```python
from build123d import *

# Parameters (mm, degrees)
SKETCH1_W                  = 101.6
SKETCH1_H                  = 177.8
BOSS_EXTRUDE1_DEPTH        = 12.7
F_10_32_TAPPED_HOLE1_D     = 4.0386
F_10_32_TAPPED_HOLE1_DEPTH = 25.4
F_10_32_TAPPED_HOLE1_TIP   = 1.213317848
SKETCH5_R                  = 12.7
SKETCH5_R_2                = 3.175
CUT_EXTRUDE1_DEPTH         = 104.175287739
SKETCH6_W                  = 61.595
SKETCH6_H                  = 61.595
CUT_EXTRUDE2_DEPTH         = 9.398
FILLET1_R                  = 3.175
SKETCH7_W                  = 67.945
SKETCH7_H                  = 67.945
CUT_EXTRUDE3_DEPTH         = 4.445
FILLET2_R                  = 3.175


with BuildPart() as part:
    # Sketch1 → Boss-Extrude1 (new body)
    with BuildSketch(Plane.XY):
        Rectangle(SKETCH1_W, SKETCH1_H)
    extrude(amount=BOSS_EXTRUDE1_DEPTH)

    # #10-32 Tapped Hole1
    with Locations(Plane(origin=(0, -88.9, 0), x_dir=(-1, 0, 0), z_dir=(0, -1, 0))):
        with Locations((31.75, -6.35), (-31.75, -6.35)):
            Hole(F_10_32_TAPPED_HOLE1_D / 2, depth=F_10_32_TAPPED_HOLE1_DEPTH)
            with Locations((0, 0, -(F_10_32_TAPPED_HOLE1_DEPTH + F_10_32_TAPPED_HOLE1_TIP / 2))):  # 118° drill point
                Cone(0, F_10_32_TAPPED_HOLE1_D / 2, F_10_32_TAPPED_HOLE1_TIP, mode=Mode.SUBTRACT)

    # Sketch5 → Cut-Extrude1 (cut, through all)
    with BuildSketch(Plane.XY.offset(12.7)):
        with Locations((0, 38.616692093)):
            Circle(SKETCH5_R)
        with Locations((-27.305, 65.921692093)):
            Circle(SKETCH5_R_2)
        with Locations((27.305, 65.921692093)):
            Circle(SKETCH5_R_2)
        with Locations((27.305, 11.311692093)):
            Circle(SKETCH5_R_2)
        with Locations((-27.305, 11.311692093)):
            Circle(SKETCH5_R_2)
    extrude(amount=-CUT_EXTRUDE1_DEPTH, mode=Mode.SUBTRACT)

    # Sketch6 → Cut-Extrude2 (cut)
    with BuildSketch(Plane(origin=(0, 0, 0), x_dir=(-1, 0, 0), z_dir=(0, 0, -1))):
        with Locations((0, 38.616692093)):
            Rectangle(SKETCH6_W, SKETCH6_H)
    extrude(amount=-CUT_EXTRUDE2_DEPTH, mode=Mode.SUBTRACT)

    # Fillet1
    fillet1_edges = [part.edges().sort_by_distance(p)[0] for p in [
        (-30.7975, 69.414192093, 4.699),
        (-30.7975, 7.819192093, 4.699),
        (30.7975, 7.819192093, 4.699),
        (30.7975, 69.414192093, 4.699),
    ]]
    fillet(fillet1_edges, radius=FILLET1_R)

    # Sketch7 → Cut-Extrude3 (cut)
    with BuildSketch(Plane(origin=(0, 0, 0), x_dir=(-1, 0, 0), z_dir=(0, 0, -1))):
        with Locations((0, 38.616692093)):
            Rectangle(SKETCH7_W, SKETCH7_H)
    extrude(amount=-CUT_EXTRUDE3_DEPTH, mode=Mode.SUBTRACT)

    # Fillet2
    fillet2_edges = [part.edges().sort_by_distance(p)[0] for p in [
        (-33.9725, 72.589192093, 2.2225),
        (-33.9725, 4.644192093, 2.2225),
        (33.9725, 4.644192093, 2.2225),
        (33.9725, 72.589192093, 2.2225),
    ]]
    fillet(fillet2_edges, radius=FILLET2_R)


solid = part.part
```
The listing builds one solid part. Answer for the finished solid, in the listing's coordinates (mm). A direction names the side the tool comes from. Round coordinates to 2 decimals unless told otherwise and drop trailing zeros. Loops run counter-clockwise (first coordinate to the right, second up) from the corner with the lowest first, then second, coordinate; pieces in that order, holes last. Notation, with made-up numbers: (-30.75, 68) - (28.25, 68) arc R10 cw to (28.25, 87) - close; hole circle Ø3 at (30.5, 88). An arc over 180 degrees is marked (long way). Use one line per item in the form item = value. Start each with the question number.
1. The part is cut by section C-C on x = 19. Determine the outline of the cut face in (y, z) (3 decimals), then the cut area to 3 significant figures.
2. The part is cut by section B-B on y = 45.5. Determine the outline of the cut face in (x, z) (1 decimal).
3. A tool of negligible diameter and unlimited length cuts with its end or side. For faces 5 (the face through (-29.89, 8.77, 6.96)), 6 (the face through (30.24, 10.1, 11.07)), 7 (the face through (-29.824, -76.022, 5.743)), from which of +Z, -Z, +X, -X, +Y, -Y can it reach the whole face along a straight path? Write none if from no direction.
4. For a pull along Y with two mould halves and no side action, classify faces 1 (the face through (-29.84, 68.51, 6.96)), 2 (the face through (-1, 1, 12.7)), 3 (the face through (0, 72.589, 2)), 4 (the face through (31.416, -62.497, 6.245)) as pulls with the +Y half, pulls with the -Y half, needs draft (parallel to the pull), parting line crosses it, or undercut.
5. Consider line 1 (X direction, y = 37.5, z = 6); line 2 (Y direction, x = 17.5, z = 4.25); line 3 (Z direction, x = 31.75, y = -74.5). Determine where each line is inside the solid, lowest interval first. Write a range as [from, to].
6. The part is cut by section A-A on x = 2. Determine the outline of the cut face in (y, z) (3 decimals).
7. Given pin 1 Ø8.5 at (x, y) = (-27.3, 11.31) entering from -Z (3 decimals); pin 2 Ø20.5 at (x, y) = (6, 35) entering from -Z, each flat-ended and moving along its own axis, determine where each tip first touches the part or whether it passes through.
Geometry check:
q1.outline = (-88.9, 0) - (4.644, 0) - (4.644, 4.445) - (7.819, 4.445) - (7.819, 9.398) - (69.414, 9.398) - (69.414, 4.445) - (72.589, 4.445) - (72.589, 0) - (88.9, 0) - (88.9, 12.7) - (-88.9, 12.7) - close
q1.area = 1,650 mm^2
q2.outline = (-50.8, 0) - (-34, 0) - (-34, 4.4) - (-30.8, 4.4) - (-30.8, 9.4) - (-10.7, 9.4) - (-10.7, 12.7) - (-50.8, 12.7) - close; (10.7, 9.4) - (30.8, 9.4) - (30.8, 4.4) - (34, 4.4) - (34, 0) - (50.8, 0) - (50.8, 12.7) - (10.7, 12.7) - close
q3.face_5 = -Z
q3.face_6 = +Z, -Z
q3.face_7 = -Y
q4.face_1 = undercut
q4.face_2 = needs draft
q4.face_3 = undercut
q4.face_4 = pulls with the -Y half
q5.line_1 = [-50.8, -30.8], [30.8, 50.8]
q5.line_2 = [-88.9, 4.64], [72.59, 88.9]
q5.line_3 = [0, 4.33], [8.37, 12.7]
q6.outline = (-88.9, 0) - (4.644, 0) - (4.644, 4.445) - (7.819, 4.445) - (7.819, 9.398) - (26.075, 9.398) - (26.075, 12.7) - (-88.9, 12.7) - close; (51.158, 9.398) - (69.414, 9.398) - (69.414, 4.445) - (72.589, 4.445) - (72.589, 0) - (88.9, 0) - (88.9, 12.7) - (51.158, 12.7) - close
q7.pin_1 = 4.445
q7.pin_2 = 9.4
